Design review of the part shown in the three views and the two pictorial views. Dimensions are in mm from the part's minimum x, y and z. A direction names the side the tool comes from. Coordinates: 2 decimals unless noted, no trailing zeros. Loops run counter-clockwise (first coordinate to the right, second up) from the corner with the lowest first, then second, coordinate; pieces in that order, holes last. Notation, with made-up numbers: (81.5, 55) -> (138.5, 55) arc R27 ccw to (138.5, 72) -> close; hole circle Ø7 at (67.5, 23). An arc over 180 degrees is marked (long way). Answer in a Markdown table with one row per item.
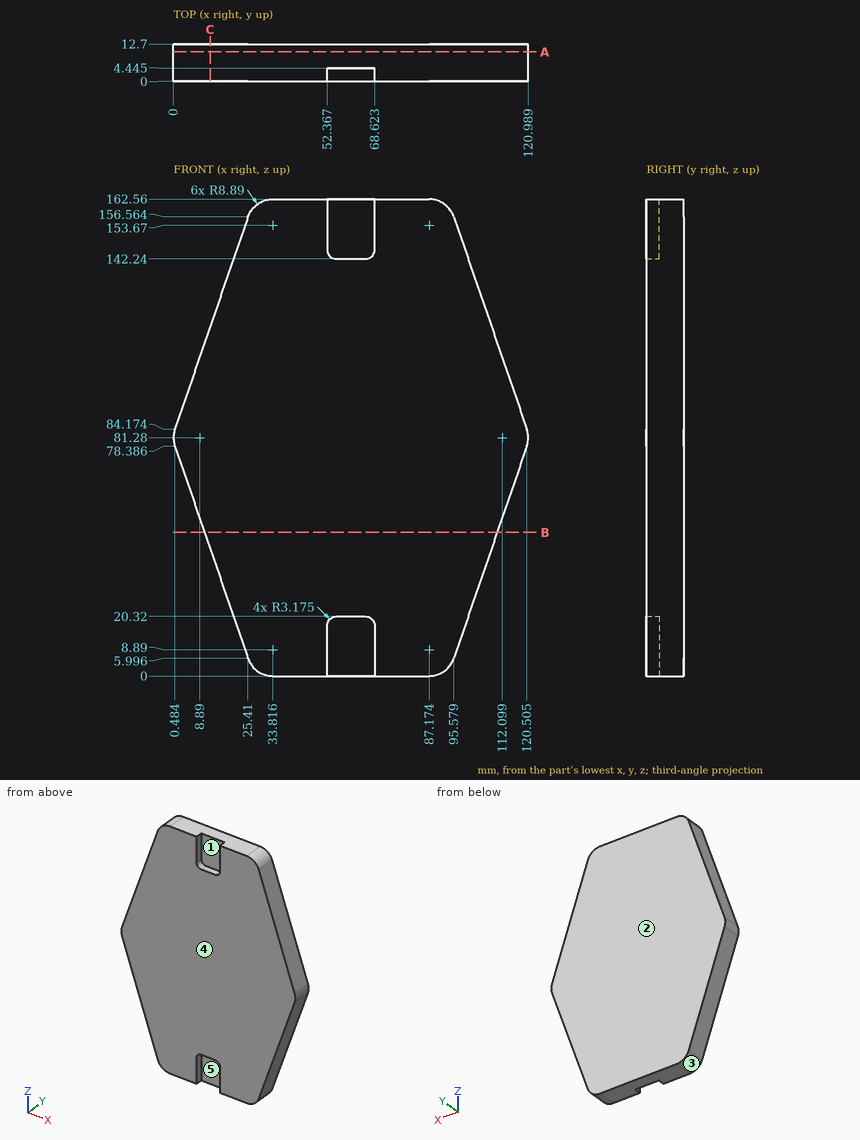
Item 1: For the marked faces 1 and 2, list the 3-axis set-ups (+Z, -Z, +X, -X, +Y, -Y) from which the entire face can be reached by the end or side of a thin tool; tool diameter is ignored.
Worked answers:
| item | result |
|---|---|
| face 1 | +Z, -Y |
| face 2 | +Z, -Z, +X, -X, +Y |
Item 2: Take a section at C-C, the plane x = 12.5. State the section outline as (y, z) points, and give its area (3 significant figures).
Worked answers:
| item | result |
|---|---|
| outline | (0, 43.49) -> (12.7, 43.49) -> (12.7, 119.07) -> (0, 119.07) -> close |
| area | 960 mm² |
Item 3: Take a section at A-A, the plane y = 10. State the section outline as (x, z) points (1 decimal).
Worked answers:
| item | result |
|---|---|
| outline | (0.5, 78.4) -> (25.4, 6) arc R8.9 ccw to (33.8, 0) -> (87.2, 0) arc R8.9 ccw to (95.6, 6) -> (120.5, 78.4) arc R8.9 ccw to (120.5, 84.2) -> (95.6, 156.6) arc R8.9 ccw to (87.2, 162.6) -> (33.8, 162.6) arc R8.9 ccw to (25.4, 156.6) -> (0.5, 84.2) arc R8.9 ccw to start |
Item 4: For L1, parallel to Z at x = 33, y = 12; L2, parallel to X at y = 4.75, z = 13; L3, parallel to X at y = 10.5, z = 62 (1 decimal), list the stretches that pass through material, from the lowest coordinate up.
Worked answers:
| item | result |
|---|---|
| L1 | 0.04 to 162.52 |
| L2 | 23 to 97.99 |
| L3 | 6.1 to 114.9 |
Item 5: Insertion check: pin 1 (1.3 mm diameter, centred on y = 3, z = 154.5, fed in from -X) (1 decimal); pin 2 (3.5 mm diameter, centred on y = 1.5, z = 11, fed in from -X) (1 decimal); pin 3 (5 mm diameter, centred on y = 3, z = 5.5, fed in from +X). Each pin has a flat end and moves straight along its axis. Give the tip position at first contact, or say it passes through.
Worked answers:
| item | result |
|---|---|
| pin 1 | x = 24.5 |
| pin 2 | x = 23.1 |
| pin 3 | x = 96.27 |
Item 6: Take a section at B-B, the plane z = 49. State the section outline as (x, y) points.
Worked answers:
| item | result |
|---|---|
| outline | (10.6, 0) -> (110.39, 0) -> (110.39, 12.7) -> (10.6, 12.7) -> close |
Item 7: The part is to be moulded in two halves that separate along X. For the marked faces 3, 4 and 5, say which applies: +X half, -X half, draft (parallel to the pull), parting line (faces both ways), or undercut.
Worked answers:
| item | result |
|---|---|
| face 3 | -X half |
| face 4 | draft |
| face 5 | undercut |
